Geometry check sheet. Reference: the model listing, model coordinates, mm. A direction names the side the tool comes from. Coordinates: 2 decimals unless noted, no trailing zeros. Order: outer loops, then holes, each group sorted by start corner. A loop starts at its lowest first (then second) coordinate and runs counter-clockwise, first axis right, second up. Notation, with made-up numbers: (-15, 9.5) - (-11, 9.5) arc R19 ccw to (-11, 20.5) - close; hole circle Ø7 at (45, 65). An arc over 180 degrees is marked (long way). Return JSON: item names as keys, results as strings. Group by question number.
Item 1: Section check C-C on y = -18. Enter the section's corners in (x, z), then the cut area to 3 significant figures.
Item 2: Section check B-B on y = 0. Enter the section's corners in (x, z), then the cut area to 3 significant figures.
Item 3: Section check A-A on x = 16. Enter the section's corners in (y, z).
Item 4: Draft check along Y on faces 1 (the flat face through (0, -9, 7)), 2 (the flat face through (-5, 11, 0)), 3 (the conical face through (-0.171, -4.132, -6.635)), 4 (the cylindrical face through (-5.44, 8.4, 0.07)). Enter one of: pulls with the +Y half, pulls with the -Y half, needs draft (parallel to the pull), parting line crosses it, or undercut.
Item 5: Section check D-D on x = 0. Enter the section's corners in (y, z), then the cut area to 4 significant figures.
Item 6: Scan lines: probe 1 along X at (y, z) = (-18.25, 0); probe 2 along Z at (x, y) = (-6, 6.75); probe 3 along X at (y, z) = (0, -3). Record each from-to range of solid material in increasing order.
Item 7: Gauge pin test, flat ends, axial feed: pin 1 (2 mm diameter, centred on y = 6, z = 0, fed in from -X); pin 2 (4.5 mm diameter, centred on y = 6.75, z = 0, fed in from +X); pin 3 (3 mm diameter, centred on x = -13, z = -2, fed in from +Y). Record the tip position at first contact, or that the pin passes through.
Item 8: Tool access check on faces 5 (the cylindrical face through (8.521, 3.333, 0.759)), 6 (the flat face through (14, -15.5, 2)), 7 (the flat face through (-0.75, 9, 0)). Record the directions out of +Z, -Z, +X, -X, +Y, -Y that give a thin tool (end or side, any length) a straight path to the whole face; none if there is none.
from build123d import *

# Parameters (mm, degrees)
BODY_DEPTH              = 7
SKETCH2_R               = 2.5
BOLT_CLEARANCE_DEPTH    = 31.858548248
SKETCH3_R               = 3.5
BOLT_HEAD_SEATING_DEPTH = 3
CLAMPING_HOLE_M4X0_7_D  = 3.3
MOUNTING_HOLE_M5X0_8_D  = 4.2
CHAMFER_2_SIZE          = 0.5


with BuildPart() as part:
    # Sketch1 → Body (new, symmetric)
    with BuildSketch(Plane.XY):
        with BuildLine():
            Line((-10, 11), (-0.75, 11))
            Line((-0.75, 11), (-0.75, 3.929058411))
            ThreePointArc((-0.75, 3.929058411), (0, -4), (0.75, 3.929058411))
            Line((0.75, 3.929058411), (0.75, 11))
            Line((0.75, 11), (10, 11))
            Line((10, 11), (10, -15.5))
            Line((10, -15.5), (21, -15.5))
            Line((21, -15.5), (21, -21.5))
            Line((21, -21.5), (-21, -21.5))
            Line((-21, -21.5), (-21, -15.5))
            Line((-21, -15.5), (-10, -15.5))
            Line((-10, -15.5), (-10, 11))
        make_face()
    extrude(amount=BODY_DEPTH, both=True)

    # Sketch2 → Bolt Clearance (cut, through all)
    with BuildSketch(Plane(origin=(0, 0, 0), x_dir=(0, 0, -1), z_dir=(1, 0, 0))):
        with Locations(Location((0, 6.75, 0), (0, 0, 180))):
            Circle(SKETCH2_R)
    extrude(amount=BOLT_CLEARANCE_DEPTH, mode=Mode.SUBTRACT)

    # Sketch3 → Bolt Head Seating (cut)
    with BuildSketch(Plane(origin=(10, 0, 0), x_dir=(0, 0, -1), z_dir=(1, 0, 0))):
        with Locations((0, 6.75)):
            Circle(SKETCH3_R)
    extrude(amount=-BOLT_HEAD_SEATING_DEPTH, mode=Mode.SUBTRACT)

    # Clamping Hole _M4x0.7 (through all)
    with Locations(Plane(origin=(-0.75, 6.75, 0), x_dir=(0, 1, 0), z_dir=(1, 0, 0))):
        with Locations((0, 0)):
            Hole(CLAMPING_HOLE_M4X0_7_D / 2)

    # Mounting Hole _M5x0.8 (through all)
    with Locations(Plane(origin=(-16, -15.5, 0), x_dir=(0, 0, 1), z_dir=(0, 1, 0))):
        with Locations((0, 0), (0, 32)):
            Hole(MOUNTING_HOLE_M5X0_8_D / 2)

    # Chamfer 2
    chamfer_2_edges = [part.edges().sort_by_distance(p)[0] for p in [
        (-21, -18.5, 7),
        (-5.375, 11, -7),
        (-0.75, 7.464529206, -7),
        (0, -4, -7),
        (0.75, 7.464529206, -7),
        (5.375, 11, -7),
        (10, -2.25, -7),
        (0, -21.5, 7),
        (15.5, -15.5, -7),
        (21, -18.5, -7),
        (0, -21.5, -7),
        (-21, -18.5, -7),
        (-15.5, -15.5, -7),
        (-10, -2.25, -7),
        (21, -18.5, 7),
        (15.5, -15.5, 7),
        (-10, 11, 0),
        (-0.75, 11, 0),
        (0.75, 11, 0),
        (10, 11, 0),
        (21, -15.5, 0),
        (21, -21.5, 0),
        (-21, -21.5, 0),
        (-21, -15.5, 0),
        (10, -2.25, 7),
        (5.375, 11, 7),
        (0.75, 7.464529206, 7),
        (0, -4, 7),
        (-0.75, 7.464529206, 7),
        (-5.375, 11, 7),
        (-10, -2.25, 7),
        (-15.5, -15.5, 7),
    ]]
    chamfer(chamfer_2_edges, length=CHAMFER_2_SIZE)


solid = part.part
Computed:
{
 "1": {"outline": "(-21, -6.5) - (-20.5, -7) - (20.5, -7) - (21, -6.5) - (21, 6.5) - (20.5, 7) - (-20.5, 7) - (-21, 6.5) - close; hole circle Ø4.2 at (-16, 0); hole circle Ø4.2 at (16, 0)", "area": "560 mm²"},
 "2": {"outline": "(-10, -6.5) - (-9.5, -7) - (-4.5, -7) - (-4, -6.5) - (-4, 6.5) - (-4.5, 7) - (-9.5, 7) - (-10, 6.5) - close; (4, -6.5) - (4.5, -7) - (9.5, -7) - (10, -6.5) - (10, 6.5) - (9.5, 7) - (4.5, 7) - (4, 6.5) - close", "area": "167 mm²"},
 "3": {"outline": "(-21.5, -6.5) - (-21, -7) - (-16, -7) - (-15.5, -6.5) - (-15.5, -2.1) - (-21.5, -2.1) - close; (-21.5, 2.1) - (-15.5, 2.1) - (-15.5, 6.5) - (-16, 7) - (-21, 7) - (-21.5, 6.5) - close"},
 "4": {"face 1": "needs draft", "face 2": "pulls with the +Y half", "face 3": "undercut", "face 4": "undercut"},
 "5": {"outline": "(-21.5, -6.5) - (-21, -7) - (-4.5, -7) - (-4, -6.5) - (-4, 6.5) - (-4.5, 7) - (-21, 7) - (-21.5, 6.5) - close", "area": "244.5 mm²"},
 "6": {"probe 1": "x = -21 to -18.1, -13.9 to 13.9, 18.1 to 21", "probe 2": "z = -7 to -1.65, 1.65 to 7", "probe 3": "x = -10 to -4, 4 to 10"},
 "7": {"pin 1": "stops at x = -10", "pin 2": "stops at x = -0.75", "pin 3": "stops at y = -15.5"},
 "8": {"face 5": "+X", "face 6": "+Z, -Z, +X, +Y", "face 7": "+Z, -Z, +Y"}
}
